```python
from build123d import *

# Parameters (mm, degrees)
F0_R     = 15.125
F1_DEPTH = 20
F2_R     = 10
F3_R     = 10


with BuildPart() as f1:
    # F0 (on Front) → F1 (new body)
    with BuildSketch(Plane.XZ):
        Polygon((0, 100), (0, 0), (150, 0), (175, 0), (75, 100), align=None)
        with Locations((37.5, 67)):
            Circle(F0_R, mode=Mode.SUBTRACT)
    extrude(amount=F1_DEPTH)

    # F2
    f2_edges = [f1.edges().sort_by_distance(p)[0] for p in [
        (0, -10, 100),
    ]]
    fillet(f2_edges, radius=F2_R)

    # F3
    f3_edges = [f1.edges().sort_by_distance(p)[0] for p in [
        (75, -10, 100),
    ]]
    fillet(f3_edges, radius=F3_R)


solid = f1.part
```
The listing builds one solid part. Answer for the finished solid, in the listing's coordinates (mm). Coordinates: 2 decimals unless noted, no trailing zeros. Write each loop counter-clockwise with the first axis right and the second up, starting at its lowest first coordinate (ties: lowest second). Pieces come first, ordered by that corner, then holes. Notation, with made-up numbers: M 24,28.5 L 65,28.5 A23 ccw 65,42.5 Z; hole C 7.5,23 d5. An arc over 180 degrees is marked long. Use a Markdown table: item, result. Add a question column.
1. Section C-C (z = 67) is taken. Give the vertices of the cut face in (x, y) (3 decimals), plus the area to 4 significant figures.
2. Given P1, Ø5, axis at y = -5, z = 41, coming from the +X side; P2, Ø1, axis at x = 134, y = -14, coming from the -Z side; P3, Ø5, axis at y = -9, z = 40.5, coming from the +X side; P4, Ø1.5, axis at y = -14.5, z = 11.5, coming from the +X side, each flat-ended and moving along its own axis, determine where each tip first touches the part or whether it passes through.
3. For a pull along Z with two mould halves and no side action, classify faces 1 (the flat face through (86, -10, 0)), 2 (the cylindrical face through (2.85, -10.14, 96.99)), 3 (the cylindrical face through (25.497, -9.86, 57.797)), 4 (the flat face through (67, 0, 40)) as +Z half, -Z half, draft (parallel to the pull), parting line (faces both ways), or undercut.
4. Section B-B (y = -12.75) is taken. Give the vertices of the cut face in (x, z) (3 decimals), plus the area to 3 significant figures.
5. Section A-A (x = 37.5) is taken. Give the vertices of the cut face in (y, z) (3 decimals).
6. Section D-D (z = 22.5) is taken. Give the vertices of the cut face in (x, y).
7. Straight lines are drawn through the part: line 1 along Z through (x, y) = (37.5, -9.25) (3 decimals); line 2 along X through (y, z) = (-5.5, 62); line 3 along Z through (x, y) = (132, -14.5). For each, find the intervals that lie inside material, in ascending order. Write a range as [from, to].
Data:
| question | item | result |
|---|---|---|
| 1 | outline | M 0,-20 L 22.375,-20 L 22.375,0 L 0,0 Z; M 52.625,-20 L 108,-20 L 108,0 L 52.625,0 Z |
| 1 | area | 1,555 mm2 |
| 2 | P1 | stops at x = 136.5 |
| 2 | P2 | stops at z = 0 |
| 2 | P3 | stops at x = 137 |
| 2 | P4 | stops at x = 164.25 |
| 3 | face 1 | -Z half |
| 3 | face 2 | +Z half |
| 3 | face 3 | undercut |
| 3 | face 4 | draft |
| 4 | outline | M 0,0 L 175,0 L 77.929,97.071 A10 ccw 70.858,100 L 10,100 A10 ccw 0,90 Z; hole C 37.5,67 d30.25 |
| 4 | area | 11,800 mm2 |
| 5 | outline | M -20,0 L 0,0 L 0,51.875 L -20,51.875 Z; M -20,82.125 L 0,82.125 L 0,100 L -20,100 Z |
| 6 | outline | M 0,-20 L 152.5,-20 L 152.5,0 L 0,0 Z |
| 7 | line 1 | z = [0, 51.875], [82.125, 100] |
| 7 | line 2 | x = [0, 23.23], [51.77, 113] |
| 7 | line 3 | z = [0, 43] |
